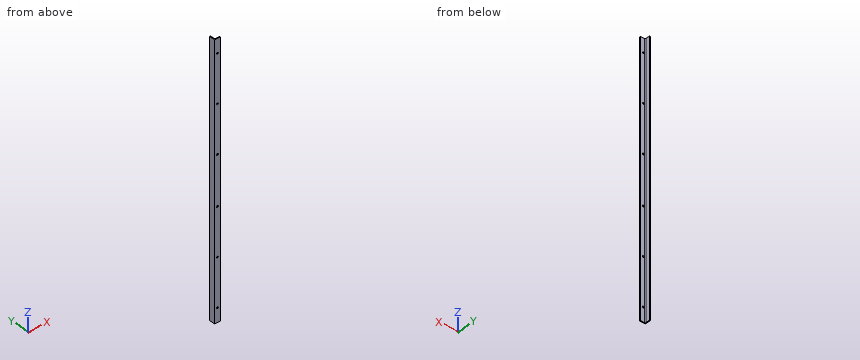
from build123d import *

# Parameters (mm, degrees)
BOSS_EXTRU_1_DEPTH      = 955
ESQUISSE2_R             = 3
ENL_V_MAT_EXTRU_1_DEPTH = 955


with BuildPart() as part:
    # Esquisse1 → Boss.-Extru.1 (new body)
    with BuildSketch(Plane.XY):
        with BuildLine():
            Line((0, 0), (0, 20))
            Line((0, 20), (3, 20))
            Line((3, 20), (3, 6))
            ThreePointArc((3, 6), (3.878679656, 3.878679656), (6, 3))
            Line((6, 3), (20, 3))
            Line((20, 3), (20, 0))
            Line((20, 0), (0, 0))
        make_face()
    extrude(amount=BOSS_EXTRU_1_DEPTH)

    # Esquisse2 → Enlèv. mat.-Extru.1 (cut)
    with BuildSketch(Plane(origin=(0, 0, 0), x_dir=(-1, 0, 0), z_dir=(0, -1, 0))):
        with Locations(Location((-10, -50, 0), (0, 0, 180))):
            Circle(ESQUISSE2_R)
        with Locations(Location((-10, -905, 0), (0, 0, 180))):
            Circle(ESQUISSE2_R)
        with Locations(Location((-10, -220, 0), (0, 0, 180))):
            Circle(ESQUISSE2_R)
        with Locations(Location((-10, -735, 0), (0, 0, 180))):
            Circle(ESQUISSE2_R)
        with Locations(Location((-10, -390, 0), (0, 0, 180))):
            Circle(ESQUISSE2_R)
        with Locations(Location((-10, -565, 0), (0, 0, 180))):
            Circle(ESQUISSE2_R)
    extrude(amount=-ENL_V_MAT_EXTRU_1_DEPTH, mode=Mode.SUBTRACT)


solid = part.part
Model file for the job. Use its own axes, mm. Give positions to 0.01 mm unless a question says otherwise; leave off trailing zeros. Loops run counter-clockwise (first coordinate to the right, second up) from the corner with the lowest first, then second, coordinate; pieces in that order, holes last. Notation, with made-up numbers: (69, 33.25) -> (93, 33.25) arc R21 cw to (93, 60.25) -> close; hole circle Ø9 at (85, -3). An arc over 180 degrees is marked (long way). Use a Markdown table: item, result. Add a question column.
(1) Wall check: line 1 along X through (y, z) = (1.65, 735); line 2 along Y through (x, z) = (8.25, 180.5). Give the ranges that are in metal, low to high.
(2) Drop flat-ended pins along their axis: pin 1 Ø7 at (y, z) = (11, 405.5) entering from +X; pin 2 Ø7 at (x, z) = (10, 905) entering from +Y. Give the stop position or say it passes through.
(3) Slice it at B-B on y = 16.25. List the corners of the cut face in (x, z), and give its area (4 significant figures).
(4) Slice it at A-A on z = 438. List the corners of the cut face in (x, y), and give its area (3 significant figures).
Filled sheet:
| question | item | result |
|---|---|---|
| 1 | line 1 | 0 to 7, 13 to 20 |
| 1 | line 2 | 0 to 3 |
| 2 | pin 1 | x = 3 |
| 2 | pin 2 | y = 3 |
| 3 | outline | (0, 0) -> (3, 0) -> (3, 955) -> (0, 955) -> close |
| 3 | area | 2,865 mm2 |
| 4 | outline | (0, 0) -> (20, 0) -> (20, 3) -> (6, 3) arc R3 cw to (3, 6) -> (3, 20) -> (0, 20) -> close |
| 4 | area | 113 mm2 |
